Work out the finished part from the listing and answer in its coordinate system (mm). Face numbers are marked on the shaded views. A direction names the side the tool comes from. Round coordinates to 2 decimals unless told otherwise and drop trailing zeros. Loops run counter-clockwise (first coordinate to the right, second up) from the corner with the lowest first, then second, coordinate; pieces in that order, holes last.
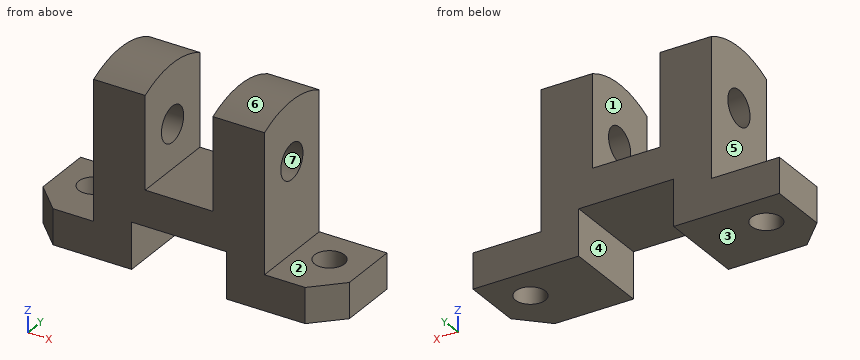
```python
from build123d import *

# Parameters (mm, degrees)
F1_DEPTH  = 32
F2_R      = 6.5
F3_DEPTH  = 19
F4_R      = 6.5
F5_DEPTH  = 19
F7_DEPTH  = 13
F8_R      = 5.5
F9_DEPTH  = 13
F11_DEPTH = 19
F13_DEPTH = 19


with BuildPart() as f1:
    # F0 (on Front) → F1 (new body)
    with BuildSketch(Plane.XZ):
        Polygon((0, 13), (0, 0), (39, 0), (39, 17), (74, 17), (74, 0), (113, 0), (113, 13), (88, 13), (88, 64.010125), (69, 64.010125), (69, 30), (44, 30), (44, 64.010125), (25, 64.010125), (25, 13), align=None)
    extrude(amount=F1_DEPTH)

    # F2 (on face) → F3 (cut, through all)
    with BuildSketch(Plane.YZ.offset(88)):
        with Locations((-16, 46)):
            Circle(F2_R)
    extrude(amount=-F3_DEPTH, mode=Mode.SUBTRACT)

    # F4 (on face) → F5 (cut, through all)
    with BuildSketch(Plane(origin=(25, 0, 0), x_dir=(0, -1, 0), z_dir=(-1, 0, 0))):
        with Locations((16, 46)):
            Circle(F4_R)
    extrude(amount=-F5_DEPTH, mode=Mode.SUBTRACT)

    # F6 (on Top) → F7 (cut, through all)
    with BuildSketch(Plane.XY):
        Polygon((0, -22), (0, -32), (10, -32), align=None)
        Polygon((113, -22), (103, -32), (113, -32), align=None)
    extrude(amount=F7_DEPTH, mode=Mode.SUBTRACT)

    # F8 (on Top) → F9 (cut, through all)
    with BuildSketch(Plane.XY):
        with Locations((13, -13)):
            Circle(F8_R)
        with Locations((100, -13)):
            Circle(F8_R)
    extrude(amount=F9_DEPTH, mode=Mode.SUBTRACT)

    # F10 (on face) → F11 (join)
    with BuildSketch(Plane.YZ.offset(88)):
        with BuildLine():
            Line((-32, 64.010125), (0, 64.010125))
            ThreePointArc((0, 64.010125), (-16, 67.88136), (-32, 64.010125))
        make_face()
    extrude(amount=-F11_DEPTH)

    # F12 (on face) → F13 (join)
    with BuildSketch(Plane(origin=(25, 0, 0), x_dir=(0, -1, 0), z_dir=(-1, 0, 0))):
        with BuildLine():
            Line((0, 64.010125), (32, 64.010125))
            ThreePointArc((32, 64.010125), (16, 67.88136), (0, 64.010125))
        make_face()
    extrude(amount=-F13_DEPTH)


solid = f1.part
```
1. Find section B-B (x = 13). Write down the section's boundary in (y, z).
Answer key:
outline: (-32, 0) - (-18.5, 0) - (-18.5, 13) - (-32, 13) - close; (-7.5, 0) - (0, 0) - (0, 13) - (-7.5, 13) - close
2. Find section C-C (z = 58). Write down the section's boundary in (x, y).
Answer key:
outline: (25, -32) - (44, -32) - (44, 0) - (25, 0) - close; (69, -32) - (88, -32) - (88, 0) - (69, 0) - close
3. Consider probe 1 along Y at (x, z) = (100, 10); probe 2 along X at (y, z) = (-25.5, 34); probe 3 along X at (y, z) = (-6.5, 3). Determine where each line is inside the solid, lowest interval first.
Answer key:
probe 1: y = -32 to -18.5, -7.5 to 0
probe 2: x = 25 to 44, 69 to 88
probe 3: x = 0 to 39, 74 to 113
4. Which of the six approach directions +Z, -Z, +X, -X, +Y, -Y give full straight-line access (tool end or side, diameter ignored) to the marked faces 1, 2, 3 and 4?
Answer key:
face 1: +Z, +Y, -Y
face 2: +Z, +X, +Y, -Y
face 3: -Z, +X, -X, +Y, -Y
face 4: -Z, +Y, -Y
5. Determine the mould class of the marked faces 5, 6 and 7 for opening direction Y: +Y half, -Y half, draft (parallel to the pull), parting line (faces both ways), or undercut.
Answer key:
face 5: draft
face 6: parting line
face 7: undercut
6. Find section D-D (y = -13). Give the number of separate pieces and of enclosed holes in the cut face, then the cut area to 3 significant figures.
Answer key:
separate pieces: 5
enclosed holes: 0
area: 2,660 mm2
7. Given pin 1 (17 mm diameter, centred on y = -16, z = 46, fed in from +X); pin 2 (12.5 mm diameter, centred on x = 60.5, y = -18, fed in from +Z); pin 3 (15 mm diameter, centred on y = -16, z = 46, fed in from -X); pin 4 (9 mm diameter, centred on x = 13, y = -13, fed in from -Z), each flat-ended and moving along its own axis, determine where each tip first touches the part or whether it passes through.
Answer key:
pin 1: stops at x = 88
pin 2: stops at z = 30
pin 3: stops at x = 25
pin 4: passes through
8. Find section A-A (z = 6). Write down the section's boundary in (x, y).
Answer key:
outline: (0, -22) - (10, -32) - (39, -32) - (39, 0) - (0, 0) - close; (74, -32) - (103, -32) - (113, -22) - (113, 0) - (74, 0) - close; hole circle Ø11 at (13, -13); hole circle Ø11 at (100, -13)
